```python
from build123d import *

# Parameters (mm, degrees)
BOSS_EXTRUDE1_DEPTH = 10
SKETCH2_R           = 2.5
CUT_EXTRUDE1_DEPTH  = 10
SKETCH3_R           = 11
CUT_EXTRUDE2_DEPTH  = 10


with BuildPart() as part:
    # Sketch1 → Boss-Extrude1 (new body)
    with BuildSketch(Plane(origin=(0, 0, 0), x_dir=(0, 0, -1), z_dir=(1, 0, 0))):
        with BuildLine():
            ThreePointArc((-209.31, 0), (0, -209.31), (209.31, 0))
            Line((209.31, 0), (-209.31, 0))
        make_face()
        with BuildLine():
            Line((-209.31, 0), (209.31, 0))
            ThreePointArc((209.31, 0), (0, 209.31), (-209.31, 0))
        make_face()
        with BuildLine():
            Line((-209.31, -224.4), (209.31, -224.4))
            Line((209.31, -224.4), (209.31, 0))
            ThreePointArc((209.31, 0), (0, -209.31), (-209.31, 0))
            Line((-209.31, 0), (-209.31, -224.4))
        make_face()
    extrude(amount=BOSS_EXTRUDE1_DEPTH)

    # Sketch2 → Cut-Extrude1 (cut)
    with BuildSketch(Plane(origin=(10, 0, 0), x_dir=(0, 0, -1), z_dir=(1, 0, 0))):
        with Locations((129.534891246, 129.534891246)):
            Circle(SKETCH2_R)
        with Locations((92.609775132, 92.609775132)):
            Circle(SKETCH2_R)
        with Locations((92.609775132, -92.609775132)):
            Circle(SKETCH2_R)
        with Locations((129.534891246, -129.534891246)):
            Circle(SKETCH2_R)
        with Locations((-92.609775132, -92.609775132)):
            Circle(SKETCH2_R)
        with Locations((-129.534891246, -129.534891246)):
            Circle(SKETCH2_R)
        with Locations((-92.609775132, 92.609775132)):
            Circle(SKETCH2_R)
        with Locations((-129.534891246, 129.534891246)):
            Circle(SKETCH2_R)
    extrude(amount=-CUT_EXTRUDE1_DEPTH, mode=Mode.SUBTRACT)

    # Sketch3 → Cut-Extrude2 (cut)
    with BuildSketch(Plane(origin=(10, 0, 0), x_dir=(0, 0, -1), z_dir=(1, 0, 0))):
        Circle(SKETCH3_R)
    extrude(amount=-CUT_EXTRUDE2_DEPTH, mode=Mode.SUBTRACT)


solid = part.part
```
For this review, take the finished solid that the model builds, in its own axes (mm). Round coordinates to 2 decimals unless told otherwise and drop trailing zeros. Write each loop counter-clockwise with the first axis right and the second up, starting at its lowest first coordinate (ties: lowest second). Pieces come first, ordered by that corner, then holes. Notation, with made-up numbers: (-26.75, 62.25) -> (31.25, 62.25) arc R28 cw to (31.25, 89.25) -> close; hole circle Ø2 at (76.25, 49). An arc over 180 degrees is marked (long way). Use one line per item in the form item = value.
Q1. Consider section B-B (x = 6.5). State how many separate pieces and enclosed holes the cut face has, then the cut area to 3 significant figures.
Resolved:
separate_pieces = 1
enclosed_holes = 9
area = 162,000 mm²
Q2. Consider section A-A (z = 0). State the section outline as (x, y) points.
Resolved:
outline = (0, -224.4) -> (10, -224.4) -> (10, -11) -> (0, -11) -> close; (0, 11) -> (10, 11) -> (10, 209.31) -> (0, 209.31) -> close
Q3. Consider section D-D (z = -111). State the section outline as (x, y) points, then the cut area to 3 significant figures.
Resolved:
outline = (0, -224.4) -> (10, -224.4) -> (10, 177.45) -> (0, 177.45) -> close
area = 4,020 mm²
Q4. Clearance check with flat-ended pins moving along their axes: pin 1 Ø8 at (y, z) = (94.5, 0.5) entering from -X; pin 2 Ø5 at (x, z) = (1.5, 56) entering from +Y. State where each tip first meets the part, or that it passes through.
Resolved:
pin_1 = 0
pin_2 = 202.36
Q5. Consider section C-C (z = -160.5). State the section outline as (x, y) points.
Resolved:
outline = (0, -224.4) -> (10, -224.4) -> (10, 134.35) -> (0, 134.35) -> close
Q6. To check wall thickness, follow probe 1 along Y at (x, z) = (3.25, 0); probe 2 along Y at (x, z) = (4.25, 131.5); probe 3 along Z at (x, y) = (7.5, -91.5). State the ranges of each line that lie inside material, in increasing order. Write a range as from..to.
Resolved:
probe_1 = -224.4..-11, 11..209.31
probe_2 = -224.4..-131.08, -127.99..127.99, 131.08..162.84
probe_3 = -209.31..-94.85, -90.37..90.37, 94.85..209.31
Q7. The part is to be moulded in two halves that separate along Z. For faces 1 (the cylindrical face through (4.93, 209.26, -4.6)), 2 (the cylindrical face through (5.07, -10.74, 2.38)), 3 (the flat face through (10, -53, 3)), 4 (the flat face through (5, -114, -209.31)), say which applies: released by +Z, released by -Z, zero draft, split by the parting line, or undercut.
Resolved:
face_1 = split by the parting line
face_2 = undercut
face_3 = zero draft
face_4 = released by -Z
